```python
from build123d import *

# Parameters (mm, degrees)
F1_DEPTH = 25.4
F2_R     = 6.985
F3_DEPTH = 25.4


with BuildPart() as f1:
    # F0 (on Front) → F1 (new body)
    with BuildSketch(Plane.XZ):
        Polygon((-34.763229, 12.741052), (-45.081979, 12.741052), (-45.081979, -7.197948), (45.088021, -7.197948), (45.088021, 5.756052), (45.088021, 6.645052), (34.769271, 6.645052), (34.769271, 5.756052), (0.003021, 5.756052), (0.003021, 11.852052), (-34.763229, 11.852052), align=None)
    extrude(amount=F1_DEPTH)

    # F2 (on face) → F3 (cut)
    with BuildSketch(Plane.XY.offset(11.852052)):
        with Locations((0.003021, -12.7)):
            Circle(F2_R)
    extrude(amount=-F3_DEPTH, mode=Mode.SUBTRACT)


solid = f1.part
```
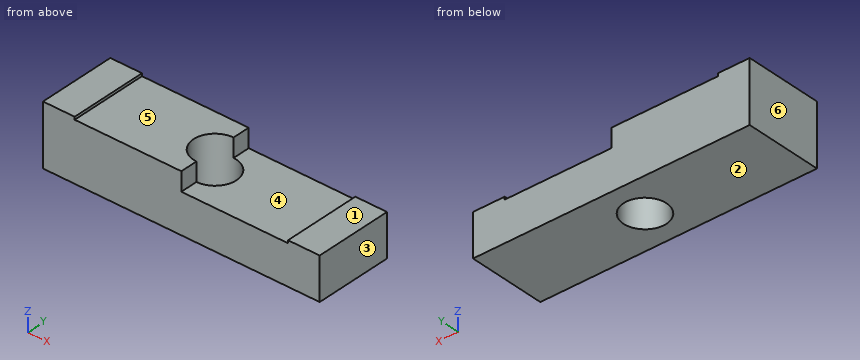
Check sheet for the modelled part. Datum: model origin and axes. Units: mm. Face numbers are marked on the shaded views. A direction names the side the tool comes from. Give positions to 0.01 mm unless a question says otherwise; leave off trailing zeros. Write each loop counter-clockwise with the first axis right and the second up, starting at its lowest first coordinate (ties: lowest second). Pieces come first, ordered by that corner, then holes. Notation, with made-up numbers: (47, 13) -> (101, 13) arc R22 ccw to (101, 23) -> close; hole circle Ø6 at (55.5, 42.25). An arc over 180 degrees is marked (long way). Use CSV: the item, a comma, the result in double quotes. Start each with the question number.
Q1. Cross-section at B-B on z = 1. Enter the section's corners in (x, y) (3 decimals), and give its area (3 significant figures).
Q2. Tool access check on the marked faces 1 and 2. Record the directions out of +Z, -Z, +X, -X, +Y, -Y that give a thin tool (end or side, any length) a straight path to the whole face; none if there is none.
Q3. Depth check by flat-ended pin: P1, Ø0.7, axis at y = -12.5, z = 12, coming from the +X side; P2, Ø2, axis at x = 23, y = -20, coming from the +Z side; P3, Ø1, axis at x = -17.5, y = -11, coming from the +Z side. Enter the tip coordinate at first touch or a pass-through.
Q4. Cross-section at C-C on x = 3. Enter the section's corners in (y, z).
Q5. Cross-section at A-A on y = -12.7. Enter the section's corners in (x, z).
Q6. Cross-section at D-D on y = -23.25. Enter the section's corners in (x, z).
Q7. Scan lines: line 1 along X through (y, z) = (-3, 6); line 2 along Z through (x, y) = (-15, -4.5); line 3 along X through (y, z) = (-12.7, -0.75). Record each from-to range of solid material in increasing order.
Q8. Release check for a two-part mould opening along X. For the marked faces 3, 4, 5 and 6 record: +X half, -X half, draft (parallel to the pull), parting line (faces both ways), or undercut.
Working result:
1,outline,"(-45.082, -25.4) -> (45.088, -25.4) -> (45.088, 0) -> (-45.082, 0) -> close; hole circle Ø13.97 at (0.003, -12.7)"
1,area,"2,140 mm^2"
2,face 1,"+Z, +X, +Y, -Y"
2,face 2,"-Z, +X, -X, +Y, -Y"
3,P1,"stops at x = -6.96"
3,P2,"stops at z = 5.76"
3,P3,"stops at z = 11.85"
4,outline,"(-25.4, -7.2) -> (-19.01, -7.2) -> (-19.01, 5.76) -> (-25.4, 5.76) -> close; (-6.39, -7.2) -> (0, -7.2) -> (0, 5.76) -> (-6.39, 5.76) -> close"
5,outline,"(-45.08, -7.2) -> (-6.98, -7.2) -> (-6.98, 11.85) -> (-34.76, 11.85) -> (-34.76, 12.74) -> (-45.08, 12.74) -> close; (6.99, -7.2) -> (45.09, -7.2) -> (45.09, 6.65) -> (34.77, 6.65) -> (34.77, 5.76) -> (6.99, 5.76) -> close"
6,outline,"(-45.08, -7.2) -> (45.09, -7.2) -> (45.09, 6.65) -> (34.77, 6.65) -> (34.77, 5.76) -> (0, 5.76) -> (0, 11.85) -> (-34.76, 11.85) -> (-34.76, 12.74) -> (-45.08, 12.74) -> close"
7,line 1,"x = -45.08 to 0, 34.77 to 45.09"
7,line 2,"z = -7.2 to 11.85"
7,line 3,"x = -45.08 to -6.98, 6.99 to 45.09"
8,face 3,"+X half"
8,face 4,"undercut"
8,face 5,"draft"
8,face 6,"-X half"
